Design review of the part built by this model. Coordinates are the model's own, in mm. Face numbers are marked on the shaded views. A direction names the side the tool comes from. Give positions to 0.01 mm unless a question says otherwise; leave off trailing zeros. Order: outer loops, then holes, each group sorted by start corner. A loop starts at its lowest first (then second) coordinate and runs counter-clockwise, first axis right, second up. Notation, with made-up numbers: (50.25, -24) -> (96.25, -24) arc R16 cw to (96.25, -3) -> close; hole circle Ø9 at (-27.75, -6). An arc over 180 degrees is marked (long way). Return JSON: item names as keys, results as strings.
```python
from build123d import *

# Parameters (mm, degrees)
F0_W = 5.8661173098
F0_H = 5.5776182562
F2_R = 2
F3_R = 2


# Not quite as in the source:
# - a feature of the source that left no trace in its solid (it failed there, or was rolled back) is left out


with BuildPart() as f1:
    # F0 (on Front) → F1 (revolve)
    with BuildSketch(Plane.XZ):
        Polygon((0, 35.7737019658), (0, 42.6976457238), (-12.7588799223, 42.6976457238), (-12.7588799223, 35.7737019658), (-5.8661173098, 35.7737019658), align=None)
        with Locations((-2.9330586549, 32.9848928377)):
            Rectangle(F0_W, F0_H)
        Polygon((0, 3.6543027963), (0, 30.1960837096), (-5.8661173098, 30.1960837096), (-14.617213048, 30.1960837096), (-14.617213048, 3.6543027963), align=None)
    revolve(axis=Axis((0, 0, 23.1759742601), (0, 0, -1)))

    # F2
    f2_edges = [f1.edges().sort_by_distance(p)[0] for p in [
        (12.75888, 0, 42.697646),
        (5.866117, 0, 30.196084),
        (14.617213, 0, 30.196084),
    ]]
    fillet(f2_edges, radius=F2_R)

    # F3
    f3_edges = [f1.edges().sort_by_distance(p)[0] for p in [
        (12.75888, 0, 35.773702),
        (14.617213, 0, 3.654303),
    ]]
    fillet(f3_edges, radius=F3_R)


solid = f1.part
```
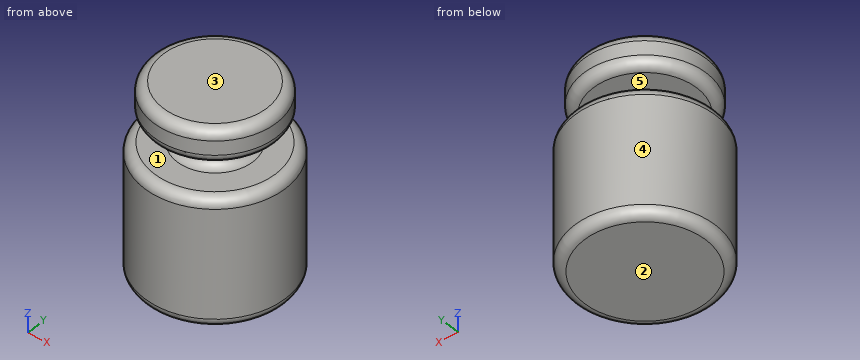
Item 1: Wall thickness on L1, parallel to Z at x = 4, y = -8.5; L2, parallel to Z at x = 0, y = 6.5; L3, parallel to X at y = -7, z = 8: over which ranges is each line inside the solid? List them lowest first. Write a range as [from, to].
Result set:
{"L1": "z = [3.65, 30.2], [35.77, 42.7]", "L2": "z = [3.65, 30.74], [35.77, 42.7]", "L3": "x = [-12.83, 12.83]"}
Item 2: Machinability: for the marked faces 4 and 5, which of the approach directions +Z, -Z, +X, -X, +Y, -Y give a long, thin tool a straight path to every point of the face, cutting with its end or side? Answer none if there is none.
Result set:
{"face 4": "+Z, -Z", "face 5": "none"}
Item 3: Add section C-C (z = 7). Give the boundary of the cut face in (x, y).
Result set:
{"outline": "circle Ø29.23 at (0, 0)"}
Item 4: Add section D-D (z = 39). Give the boundary of the cut face in (x, y).
Result set:
{"outline": "circle Ø25.52 at (0, 0)"}
Item 5: For pin 1 (12 mm diameter, centred on x = -8.5, z = 27.5, fed in from +Y); pin 2 (3 mm diameter, centred on y = -11, z = 16, fed in from -X); pin 3 (1.5 mm diameter, centred on x = 9.5, z = 16, fed in from +Y), all flat-tipped, find the tip position at first contact; note any pin that passes through.
Result set:
{"pin 1": "stops at y = 14.4", "pin 2": "stops at x = -11.11", "pin 3": "stops at y = 11.71"}
Item 6: Add section A-A (y = 0). Give the boundary of the cut face in (x, z).
Result set:
{"outline": "(-14.62, 5.65) arc R2 ccw to (-12.62, 3.65) -> (12.62, 3.65) arc R2 ccw to (14.62, 5.65) -> (14.62, 28.2) arc R2 ccw to (12.62, 30.2) -> (7.87, 30.2) arc R2 cw to (5.87, 32.2) -> (5.87, 35.77) -> (10.76, 35.77) arc R2 ccw to (12.76, 37.77) -> (12.76, 40.7) arc R2 ccw to (10.76, 42.7) -> (-10.76, 42.7) arc R2 ccw to (-12.76, 40.7) -> (-12.76, 37.77) arc R2 ccw to (-10.76, 35.77) -> (-5.87, 35.77) -> (-5.87, 32.2) arc R2 cw to (-7.87, 30.2) -> (-12.62, 30.2) arc R2 ccw to (-14.62, 28.2) -> close"}
Item 7: Mouldability with a two-part tool opening along Z and no side actions: class the marked faces 1, 2 and 3 as released by +Z, released by -Z, zero draft, split by the parting line, or undercut.
Result set:
{"face 1": "undercut", "face 2": "released by -Z", "face 3": "released by +Z"}
